For this review, use the dimensioned drawing (mm, ordinates from the lowest corner) and the shaded views. Coordinates: 2 decimals unless noted, no trailing zeros. Write each loop counter-clockwise with the first axis right and the second up, starting at its lowest first coordinate (ties: lowest second). Pieces come first, ordered by that corner, then holes. Notation, with made-up numbers: (70.25, -2.5) - (118.25, -2.5) arc R28 ccw to (118.25, 29.5) - close; hole circle Ø7 at (17, 59). An arc over 180 degrees is marked (long way). One line per item, written item: value.
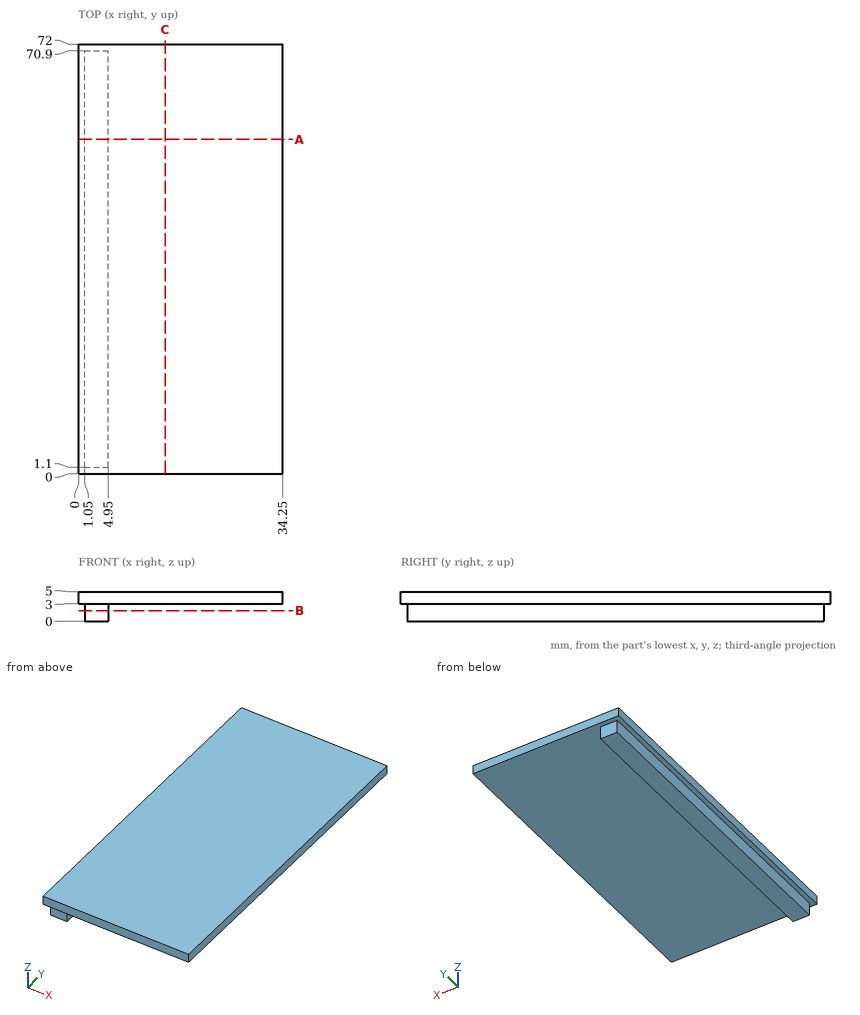
1. Consider section C-C, the plane x = 14.5. Write out the cut boundary in (y, z), then the cut area to 3 significant figures.
Answer block:
outline: (0, 3) - (72, 3) - (72, 5) - (0, 5) - close
area: 144 mm^2
2. Consider section A-A, the plane y = 56. Write out the cut boundary in (x, z), then the cut area to 3 significant figures.
Answer block:
outline: (0, 3) - (1.05, 3) - (1.05, 0) - (4.95, 0) - (4.95, 3) - (34.25, 3) - (34.25, 5) - (0, 5) - close
area: 80.2 mm^2
3. Consider section B-B, the plane z = 1.8. Write out the cut boundary in (x, y).
Answer block:
outline: (1.05, 1.1) - (4.95, 1.1) - (4.95, 70.9) - (1.05, 70.9) - close
4. Wall thickness on line 1 along Z through (x, y) = (22.5, 23.5); line 2 along X through (y, z) = (37.5, 1.95); line 3 along Y through (x, z) = (4.5, 1.95): over which ranges is each line inside the solid? List them lowest first.
Answer block:
line 1: z = 3 to 5
line 2: x = 1.05 to 4.95
line 3: y = 1.1 to 70.9
5. Insertion check: pin 1 Ø1 at (y, z) = (26, 1) entering from +X; pin 2 Ø1.5 at (x, z) = (3, 1.5) entering from -Y; pin 3 Ø4 at (x, y) = (15.5, 9.5) entering from -Z. Each pin has a flat end and moves straight along its axis. Give the tip position at first contact, or say it passes through.
Answer block:
pin 1: stops at x = 4.95
pin 2: stops at y = 1.1
pin 3: stops at z = 3
